Here's the drawing with two shaded views (mm, measured from the low corner). I have some questions. Round coordinates to 2 decimals unless told otherwise and drop trailing zeros. Order: outer loops, then holes, each group sorted by start corner. A loop starts at its lowest first (then second) coordinate and runs counter-clockwise, first axis right, second up. Notation, with made-up numbers: M -11,20 L 13,20 A17 ccw 13,44 Z; hole C 51.5,46.25 d10. An arc over 180 degrees is marked long. One line per question, with ' | ' between items.
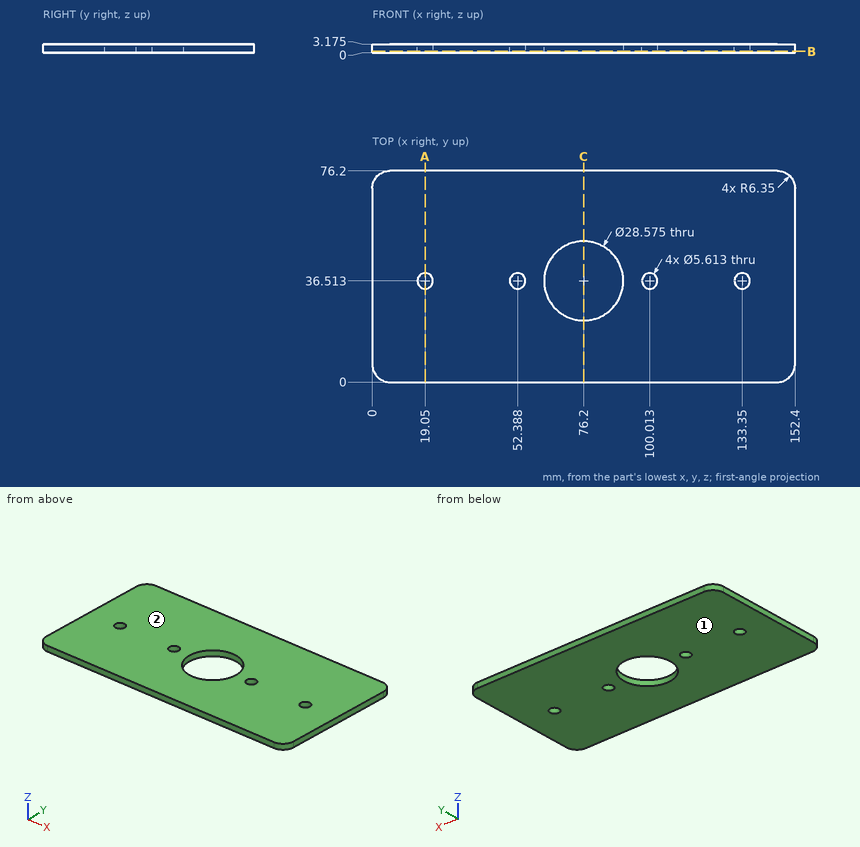
(1) Thinking about a two-plate mould opening in Z: for the marked faces 1 and 2, which applies, released by +Z, released by -Z, zero draft, split by the parting line, or undercut?
Final values:
face 1: released by -Z | face 2: released by +Z
(2) If we section it at C-C on x = 76.2: Please give me the cut outline in (y, z) (1 decimal).
Final values:
outline: M 0,0 L 22.2,0 L 22.2,3.2 L 0,3.2 Z; M 50.8,0 L 76.2,0 L 76.2,3.2 L 50.8,3.2 Z
(3) Please list where these lines run through material, in increasing order: probe 1 along Y at (x, z) = (75.5, 0.75); probe 2 along Y at (x, z) = (71, 1.85) (1 decimal); probe 3 along X at (y, z) = (28, 0.45) (1 decimal). Write a range as [from, to].
Final values:
probe 1: [0, 22.24], [50.78, 76.2] | probe 2: [0, 23.2], [49.8, 76.2] | probe 3: [0, 64.7], [87.7, 152.4]
(4) If we section it at A-A on x = 19.05: Please give me the cut outline in (y, z) (1 decimal).
Final values:
outline: M 0,0 L 33.7,0 L 33.7,3.2 L 0,3.2 Z; M 39.3,0 L 76.2,0 L 76.2,3.2 L 39.3,3.2 Z
(5) If we section it at B-B on z = 0.5: State how many separate pieces and enclosed holes the cut face has, plus the area to 3 significant figures.
Final values:
separate pieces: 1 | enclosed holes: 5 | area: 10,800 mm^2
